Source: CAD feature listing. Evaluate the final solid. Frame: model axes, mm. A direction names the side the tool comes from. Coordinates: 2 decimals unless noted, no trailing zeros. Write each loop counter-clockwise with the first axis right and the second up, starting at its lowest first coordinate (ties: lowest second). Pieces come first, ordered by that corner, then holes. Notation, with made-up numbers: (-39, 24) -> (-29, 24) arc R26 cw to (-29, 51) -> close; hole circle Ø5 at (-26.75, -5.5). An arc over 180 degrees is marked (long way). Write item = value, one per line.
from build123d import *

# Parameters (mm, degrees)
F0_R     = 1
F0_R_2   = 1.4
F1_DEPTH = 3


with BuildPart() as f1:
    # F0 (on Front) → F1 (new body)
    with BuildSketch(Plane.XZ):
        Polygon((66.201438, -33.121341), (62.964357, -34.452247), (62.260879, -32.741219), (67.347719, -30.649795), (66.663254, -28.985011), (61.576413, -31.076434), (60.872934, -29.365406), (64.110014, -28.0345), (65.959775, -27.273983), (65.199257, -25.424222), (64.016773, -16.131517), (64.31804, -14.154337), (62.340861, -13.85307), (58.880797, -13.325852), (59.159469, -11.496961), (64.596712, -12.325446), (64.867853, -10.545985), (59.43061, -9.7175), (59.709282, -7.888609), (60.945019, -8.076901), (63.169346, -8.415827), (65.146525, -8.717094), (67.975146, -9.148098), (67.975146, -7.125014), (65.447792, -6.739915), (61.246286, -6.099722), (57.04478, -5.459529), (55.613761, -14.851131), (57.337776, -28.656422), (60.113665, -35.408047), (57.337776, -36.549337), (57.337776, -41.735669), (67.975146, -41.735669), (67.975146, -32.392092), align=None)
        with Locations((63.074746, -39.142503)):
            Circle(F0_R, mode=Mode.SUBTRACT)
        with Locations((60.54433, -21.285346)):
            Circle(F0_R_2, mode=Mode.SUBTRACT)
    extrude(amount=F1_DEPTH)


solid = f1.part
1) Cut plane A-A, the plane z = -38.5. Output: boundary loops of the cut face in (x, y), and give its area (3 significant figures).
Answer block:
outline = (57.34, -3) -> (62.31, -3) -> (62.31, 0) -> (57.34, 0) -> close; (63.84, -3) -> (67.98, -3) -> (67.98, 0) -> (63.84, 0) -> close
area = 27.3 mm2
2) Cut plane B-B, the plane x = 58.5. Output: boundary loops of the cut face in (y, z).
Answer block:
outline = (-3, -41.74) -> (0, -41.74) -> (0, -36.07) -> (-3, -36.07) -> close; (-3, -31.48) -> (0, -31.48) -> (0, -5.68) -> (-3, -5.68) -> close
3) Material intervals for probe 1 along Z at (x, y) = (62, -0.65); probe 2 along Z at (x, y) = (61, -2.45); probe 3 along X at (y, z) = (-0.6, -30), sorted ascending. Write a range as [from, to].
Answer block:
probe_1 = [-41.74, -30.9], [-28.9, -13.8], [-11.93, -10.11], [-8.24, -6.21]
probe_2 = [-41.74, -29.67], [-29.31, -22.61], [-19.96, -13.65], [-11.78, -9.96], [-8.09, -6.06]
probe_3 = [57.89, 61.13], [64.19, 67.08]
4) First-contact query: pin 1 Ø0.9 at (y, z) = (-2, -40.5) entering from -X; pin 2 Ø1.6 at (x, z) = (63.07, -39.14) entering from +Y; pin 3 Ø1 at (x, y) = (66, -1) entering from +Z. Flat tips, straight axial feed; report the tip coordinate or a pass-through.
Answer block:
pin_1 = 57.34
pin_2 = through
pin_3 = -6.75
5) Reachability of faces 1 (the flat face through (65.6, -1.5, -26.4)), 2 (the flat face through (64.155, -1.479, -30.016)), 3 (the flat face through (57.338, -1, -39)), 4 (the flat face through (58.75, -1.48, -35.97)), 5 (the flat face through (67.975, -1, -37)) from +Z, -Z, +X, -X, +Y, -Y: full face, straight path, thin tool, end or side. Return the list, or none.
Answer block:
face_1 = +X, +Y, -Y
face_2 = +Y, -Y
face_3 = -Z, -X, +Y, -Y
face_4 = -X, +Y, -Y
face_5 = +Z, -Z, +X, +Y, -Y
6) Cut plane D-D, the plane z = -24. Output: boundary loops of the cut face in (x, y).
Answer block:
outline = (56.76, -3) -> (65.02, -3) -> (65.02, 0) -> (56.76, 0) -> close
7) Pull-direction query (Z, two-part tool) for faces 6 (the flat face through (64.616, -1.479, -20.843)), 7 (the flat face through (62, -3, -23)), 8 (the flat face through (56.464, -1.479, -21.657)); classes: +Z half, -Z half, draft (parallel to the pull), parting line (faces both ways), or undercut.
Answer block:
face_6 = undercut
face_7 = draft
face_8 = -Z half
8) Cut plane C-C, the plane y = -0.4. Give the number of separate pieces and of enclosed holes in the cut face, and give its area (3 significant figures).
Answer block:
separate_pieces = 1
enclosed_holes = 2
area = 272 mm2
